Check sheet for the drawn part. Datum: minimum x, y, z corner. Units: mm. A direction names the side the tool comes from. Round coordinates to 2 decimals unless told otherwise and drop trailing zeros. Loops run counter-clockwise (first coordinate to the right, second up) from the corner with the lowest first, then second, coordinate; pieces in that order, holes last. Notation, with made-up numbers: (0, 58.25) -> (24, 58.25) arc R8 cw to (24, 72.25) -> close; hole circle Ø6 at (-18, 58.5). An arc over 180 degrees is marked (long way). Return JSON: item names as keys, results as strings.
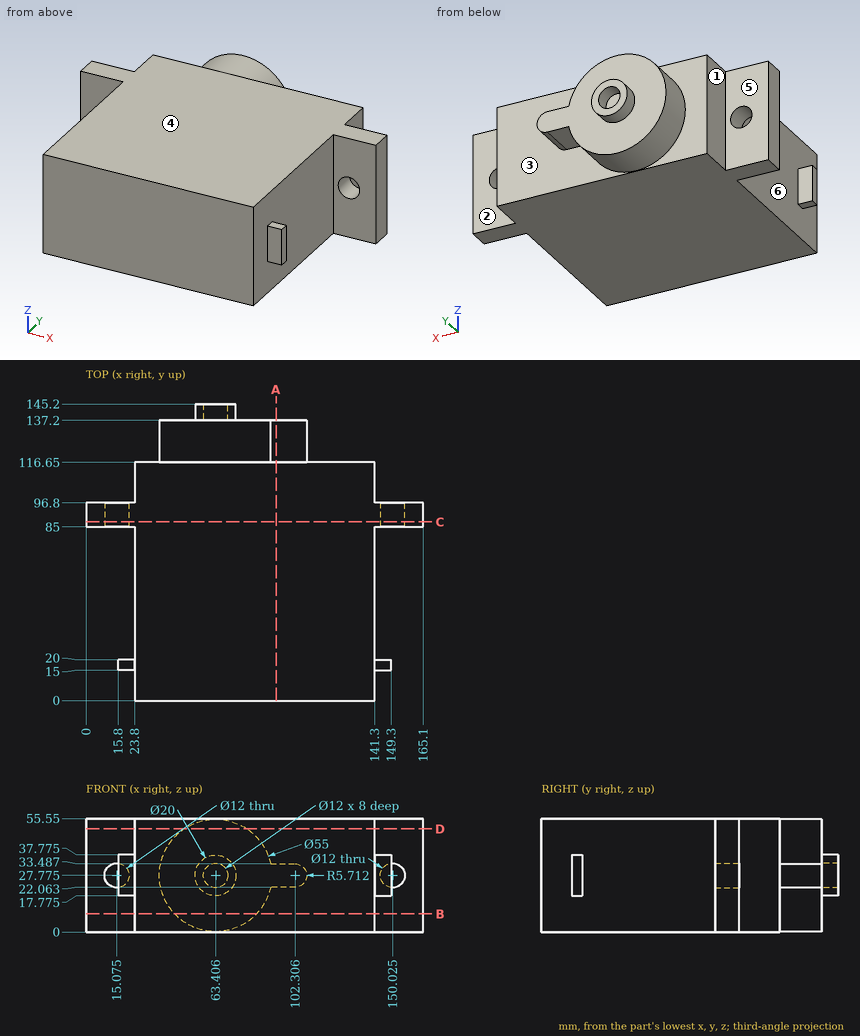
Q1. Section check D-D (z = 50.5). Record the boundary of the cut face in (x, y), then the cut area to 3 significant figures.
Results list:
{"outline": "(0, 85) -> (23.8, 85) -> (23.8, 0) -> (141.3, 0) -> (141.3, 85) -> (165.1, 85) -> (165.1, 96.8) -> (141.3, 96.8) -> (141.3, 116.65) -> (78.89, 116.65) -> (78.89, 137.2) -> (47.92, 137.2) -> (47.92, 116.65) -> (23.8, 116.65) -> (23.8, 96.8) -> (0, 96.8) -> close", "area": "14,900 mm^2"}
Q2. Section check C-C (y = 87.5). Count the separate pieces of the cut face and the enclosed holes in it.
Results list:
{"separate pieces": "1", "enclosed holes": "2"}
Q3. Draft check along Y on the marked faces 4, 5 and 6. Enter one of: released by +Y, released by -Y, zero draft, split by the parting line, or undercut.
Results list:
{"face 4": "zero draft", "face 5": "released by +Y", "face 6": "undercut"}
Q4. Go/stop test with flat-tipped pins: pin 1 (4 mm diameter, centred on x = 21, z = 24, fed in from +Y); pin 2 (1 mm diameter, centred on x = 48.5, z = 44, fed in from +Y); pin 3 (10 mm diameter, centred on y = 106.5, z = 18, fed in from -X). Record where each tip stops, or that it passes through.
Results list:
{"pin 1": "y = 96.8", "pin 2": "y = 137.2", "pin 3": "x = 23.8"}
Q5. Section check B-B (z = 9). Record the boundary of the cut face in (x, y).
Results list:
{"outline": "(0, 85) -> (23.8, 85) -> (23.8, 0) -> (141.3, 0) -> (141.3, 85) -> (165.1, 85) -> (165.1, 96.8) -> (141.3, 96.8) -> (141.3, 116.65) -> (83.5, 116.65) -> (83.5, 137.2) -> (43.31, 137.2) -> (43.31, 116.65) -> (23.8, 116.65) -> (23.8, 96.8) -> (0, 96.8) -> close"}
Q6. Section check A-A (x = 93). Record the boundary of the cut face in (y, z).
Results list:
{"outline": "(0, 0) -> (116.65, 0) -> (116.65, 22.06) -> (137.2, 22.06) -> (137.2, 33.49) -> (116.65, 33.49) -> (116.65, 55.55) -> (0, 55.55) -> close"}
Q7. Tool access check on the marked faces 1, 2 and 3. Record the directions out of +Z, -Z, +X, -X, +Y, -Y that give a thin tool (end or side, any length) a straight path to the whole face; none if there is none.
Results list:
{"face 1": "+Z, -Z, -X, +Y", "face 2": "+Z, -Z, +X, +Y", "face 3": "+Y"}
Q8. Material ranges on line 1 (Y direction, x = 20, z = 33); line 2 (Y direction, x = 14.5, z = 39); line 3 (X direction, y = 70, z = 35), recorded low to high.
Results list:
{"line 1": "15 to 20, 85 to 96.8", "line 2": "85 to 96.8", "line 3": "23.8 to 141.3"}
